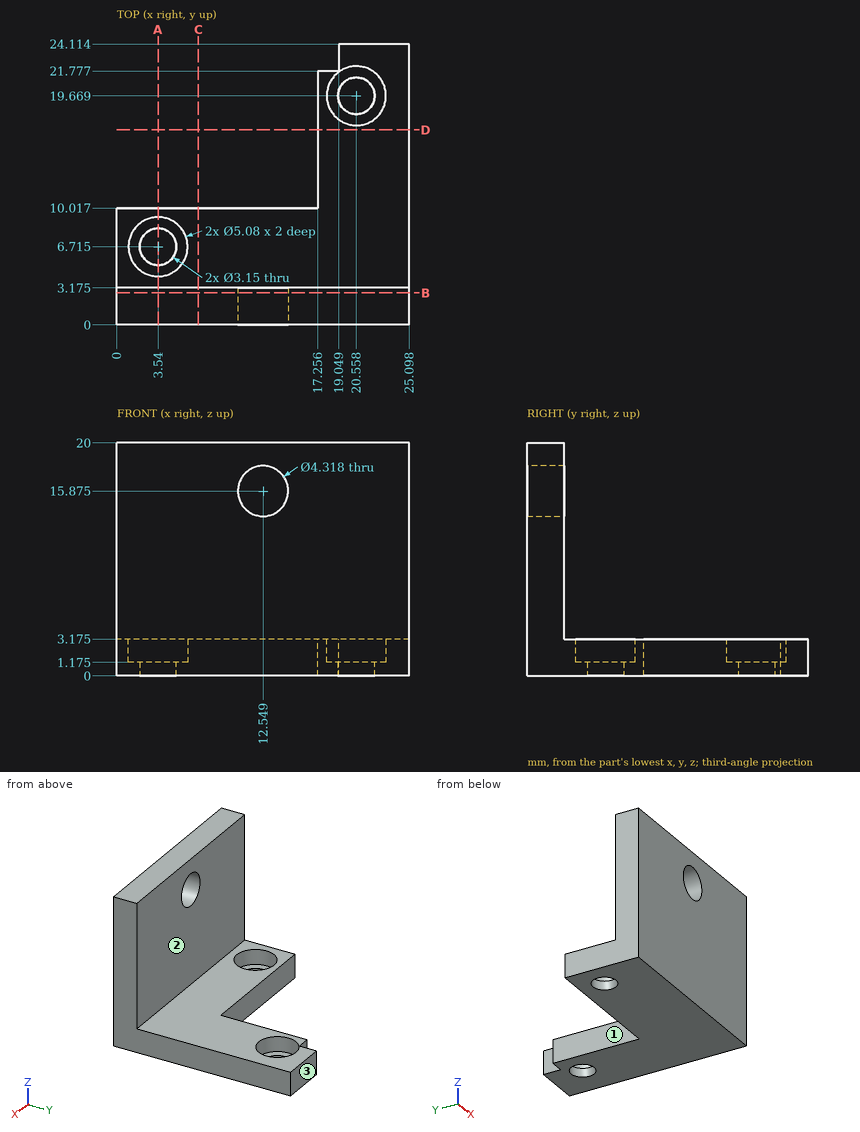
Source: three-view drawing plus pictorial views. Frame: mm from the lowest corner of the part. A direction names the side the tool comes from. Coordinates: 2 decimals unless noted, no trailing zeros. Loops run counter-clockwise (first coordinate to the right, second up) from the corner with the lowest first, then second, coordinate; pieces in that order, holes last. Notation, with made-up numbers: (87.25, -39.5) - (115.25, -39.5) arc R7 cw to (115.25, -29.5) - close; hole circle Ø4 at (-23, -10.75). An arc over 180 degrees is marked (long way). Answer in a Markdown table with one row per item. Add a question column.
Item 1: Section query C-C on x = 7. Return the cut outline in (y, z) (1 decimal).
Item 2: Section query D-D on y = 16.75. Return the cut outline in (x, z) (1 decimal).
Item 3: Section query A-A on x = 3.54. Return the cut outline in (y, z) (1 decimal).
Item 4: Section query B-B on y = 2.75. Return the cut outline in (x, z) (1 decimal).
Item 5: Access query for the marked faces 1, 2 and 3. Directions: +Z, -Z, +X, -X, +Y, -Y. A direction counts if a zero-diameter tool reaches every point of the face in a straight line with its end or side. Return the directions, or none.
Item 6: Line query: line 1 along Y through (x, z) = (3.54, 2.4) (1 decimal); line 2 along Y through (x, z) = (3.54, 0.6); line 3 along Y through (x, z) = (6.5, 15.75) (1 decimal). Output: solid intervals per line, ascending. Write a range as [from, to].
Item 7: Contact query for flat-ended pins moving along their axis: P1, Ø3, axis at x = 4, y = 11, coming from the +Z side (3 decimals); P2, Ø1.5, axis at x = 16.5, z = 16, coming from the +Y side (3 decimals); P3, Ø3.5, axis at x = 10, z = 2, coming from the +Y side. Output: stop coordinate, or through.
Recorded:
| question | item | result |
|---|---|---|
| 1 | outline | (0, 0) - (10, 0) - (10, 3.2) - (3.2, 3.2) - (3.2, 20) - (0, 20) - close |
| 2 | outline | (17.3, 0) - (25.1, 0) - (25.1, 3.2) - (17.3, 3.2) - close |
| 3 | outline | (0, 0) - (5.1, 0) - (5.1, 1.2) - (4.2, 1.2) - (4.2, 3.2) - (3.2, 3.2) - (3.2, 20) - (0, 20) - close; (8.3, 0) - (10, 0) - (10, 3.2) - (9.3, 3.2) - (9.3, 1.2) - (8.3, 1.2) - close |
| 4 | outline | (0, 0) - (25.1, 0) - (25.1, 20) - (0, 20) - close; hole circle Ø4.3 at (12.5, 15.9) |
| 5 | face 1 | +Z, -Z, -X, +Y |
| 5 | face 2 | +Z, +X, -X, +Y |
| 5 | face 3 | +Z, -Z, +X, -X, +Y |
| 6 | line 1 | [0, 4.2], [9.3, 10] |
| 6 | line 2 | [0, 5.14], [8.29, 10.02] |
| 6 | line 3 | [0, 3.2] |
| 7 | P1 | z = 3.175 |
| 7 | P2 | y = 3.175 |
| 7 | P3 | y = 10.02 |
